For this review, take the finished solid that the model builds, in its own axes (mm). Face numbers are marked on the shaded views. A direction names the side the tool comes from. Coordinates: 2 decimals unless noted, no trailing zeros. Write each loop counter-clockwise with the first axis right and the second up, starting at its lowest first coordinate (ties: lowest second). Pieces come first, ordered by that corner, then holes. Notation, with made-up numbers: (-3.75, -29.75) -> (29.25, -29.75) arc R11 ccw to (29.25, -25.75) -> close; hole circle Ø9 at (-8, 59). An arc over 180 degrees is marked (long way). One line per item, written item: value. Start each with the question number.
1) Add section A-A (x = 0). State the section outline as (y, z) points, and give its area (3 significant figures).
2) Add section B-B (z = 0). State the section outline as (x, y) points, and give its area (3 significant figures).
3) Mouldability with a two-part tool opening along X and no side actions: class the marked faces 1, 2 and 3 as released by +X, released by -X, zero draft, split by the parting line, or undercut.
4) Machinability: for the marked faces 4, 5 and 6, which of the approach directions +Z, -Z, +X, -X, +Y, -Y give a long, thin tool a straight path to every point of the face, cutting with its end or side? Answer none if there is none.
5) For probe 1 along Z at (x, y) = (0, 30); probe 2 along Z at (x, y) = (49, 78); probe 3 along X at (y, z) = (33, -23), list the stretches that pass through material, from the lowest coordinate up. Write a range as from..to.
6) For pin 1 Ø6 at (y, z) = (63, -11.5) entering from -X; pin 2 Ø16.5 at (x, y) = (57.5, 88.5) entering from -Z; pin 3 Ø16.5 at (x, z) = (55.5, -9) entering from -Y, all flat-tipped, find the tip position at first contact; note any pin that passes through.
7) Add section D-D (x = 16.5). State the section outline as (y, z) points.
8) Add section C-C (y = 39.5). State the section outline as (x, z) points.
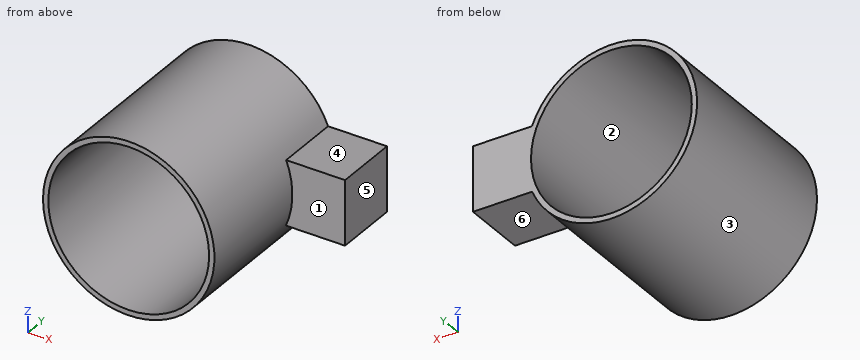
Autodesk Inventor part; units mm, degrees
ref_plane "YZ Plane" through (0, 0, 0) normal (1, 0, 0) x (0, 1, 0)
ref_plane "XZ Plane" through (0, 0, 0) normal (0, 1, 0) x (-1, 0, 0)
ref_plane "XY Plane" through (0, 0, 0) normal (0, 0, 1) x (1, 0, 0)
sketch "Sketch13" plane through (0, 0, 0) normal (0, 1, 0) x (-1, 0, 0)
  circle A0 centre (0, 0) radius 44.2659
  circle A1 centre (0, 0) radius 47.1927
  dimension "d24" = 88.5317
extrude "Extrusion7" add sketch "Sketch13" along normal blind 101.6
sketch "Sketch14" plane through (0, 101.6, 0) normal (0, 1, 0) x (1, 0, 0)
  line L0 (43.6505, 17.9383) -> (76.2, 17.9383)
  line L1 (76.2, 17.9383) -> (76.2, -17.6217)
  line L2 (76.2, -17.6217) -> (43.7793, -17.6217)
  circle A0 centre (0, 0) radius 47.1927
  arc A1 (43.7793, -17.6217) -> (43.6505, 17.9383) centre (0, 0) ccw
  dimension "d29" = 35.56
extrude "Extrusion8" add sketch "Sketch14" against normal blind 35.56 contours L0 L1 L2 A0
properties part number "cock storage holder" material "Stainless Steel"
Numbers:
1. outline: (0, -47.19) -> (101.6, -47.19) -> (101.6, -44.27) -> (0, -44.27) -> close; (0, 44.27) -> (101.6, 44.27) -> (101.6, 47.19) -> (0, 47.19) -> close
1. area: 595 mm²
2. outline: (-47.19, 0) -> (-44.27, 0) -> (-44.27, 101.6) -> (-47.19, 101.6) -> close; (44.27, 0) -> (47.19, 0) -> (47.19, 66.04) -> (76.2, 66.04) -> (76.2, 101.6) -> (44.27, 101.6) -> close
2. area: 1,630 mm²
3. face 1: zero draft
3. face 2: undercut
3. face 3: split by the parting line
4. face 4: +Z, +X, +Y, -Y
4. face 5: +Z, -Z, +X, +Y, -Y
4. face 6: -Z, +X, +Y, -Y
5. probe 1: -47.19..-44.27, 44.27..47.19
5. probe 2: -17.94..17.62
5. probe 3: -41.21..-37.82, 37.82..41.21
6. pin 1: x = -46.42
6. pin 2: z = -17.94
6. pin 3: y = 66.04
7. outline: (0, -44.21) -> (101.6, -44.21) -> (101.6, -41.08) -> (0, -41.08) -> close; (0, 41.08) -> (101.6, 41.08) -> (101.6, 44.21) -> (0, 44.21) -> close
8. outline: circle Ø94.39 at (0, 0); hole circle Ø88.53 at (0, 0)
